Autodesk Inventor part; units mm, degrees
ref_plane "YZ Plane" through (0, 0, 0) normal (1, 0, 0) x (0, 1, 0)
ref_plane "XZ Plane" through (0, 0, 0) normal (0, 1, 0) x (-1, 0, 0)
ref_plane "XY Plane" through (0, 0, 0) normal (0, 0, 1) x (1, 0, 0)
sketch "Sketch1" plane through (0, 0, 0) normal (0, 0, 1) x (1, 0, 0)
  line L0 (-43.38, 0) -> (7.23, 0) construction
  line L1 (0, -97.41) -> (0, 25.51)
  line L2 (0, 7.95) -> (-31.775, 7.95)
  line L3 (-31.775, 7.95) -> (-31.775, 3.5363)
  line L4 (-31.775, 3.5363) -> (-28.125, 1.4289)
  line L5 (-28.125, 1.4289) -> (-28.125, -1.4289)
  line L6 (-31.775, -7.95) -> (0, -7.95)
  line L7 (-28.125, -1.4289) -> (-31.775, -3.5363)
  line L8 (-31.775, -3.5363) -> (-31.775, -7.95)
  circle A0 centre (-32.65, 0) radius 3.5 construction
  line L9 (-22.225, -7.95) -> (-22.225, -11.45)
  line L10 (-22.225, -11.45) -> (0, -11.45) construction
  line L11 (-22.225, -11.45) -> (-12.2465, -79.85)
  line L12 (-12.2465, -79.85) -> (-8, -79.85)
  line L13 (-8, -79.85) -> (-8, -54.85)
  line L14 (-8, -54.85) -> (0, -54.85)
  point P0 (0, 0)
  point P1 (-36.15, 0)
  dimension "d5" = 7
  dimension "d0" = 60
  dimension "d1" = 56.25
  dimension "d2" = 63.55
  dimension "d3" = 15.9
  dimension "d6" = 72.3
  dimension "d14" = 3.5
  dimension "d15" = 44.45
  dimension "d16" = 68.4
  dimension "d17" = 8.3
  dimension "d18" = 25
  dimension "d19" = 16
  dimension "d20" = 24.493
revolve "Revolution1" add sketch "Sketch1" angle 360 about axis through (0, -10, 0) along (0, 1, 0)
sketch "Sketch2" plane through (0, 7.95, 0) normal (0, 1, 0) x (1, 0, 0)
  circle A0 centre (0, 0) radius 31.775 construction
  line L0 (-44.485, 0) -> (44.485, 0) construction
  line L1 (0, 44.485) -> (0, -44.485) construction
  line L2 (-31.775, 8.05) -> (-23.825, 8.05)
  line L3 (-23.825, 8.05) -> (-23.825, -8.05)
  line L4 (-23.825, -8.05) -> (-31.775, -8.05)
  line L5 (-31.775, -8.05) -> (-31.775, 8.05)
  circle A1 centre (0, 0) radius 31.775
  line L6 (31.775, 8.05) -> (23.825, 8.05)
  line L7 (23.825, 8.05) -> (23.825, -8.05)
  line L8 (23.825, -8.05) -> (31.775, -8.05)
  line L9 (31.775, -8.05) -> (31.775, 8.05)
  point P0 (-31.775, 0)
  point P1 (31.775, 0)
  point P2 (30.7384, -8.05)
  point P3 (30.7384, 8.05)
  point P4 (-30.7384, 8.05)
  point P5 (-30.7384, -8.05)
  dimension "d12" = 16.1
  dimension "d13" = 47.65
extrude "Extrusion1" cut sketch "Sketch2" against normal through all contours L2 L3 L4 A1 | A1 L8 L7 L6
properties part number "SK40Collar"
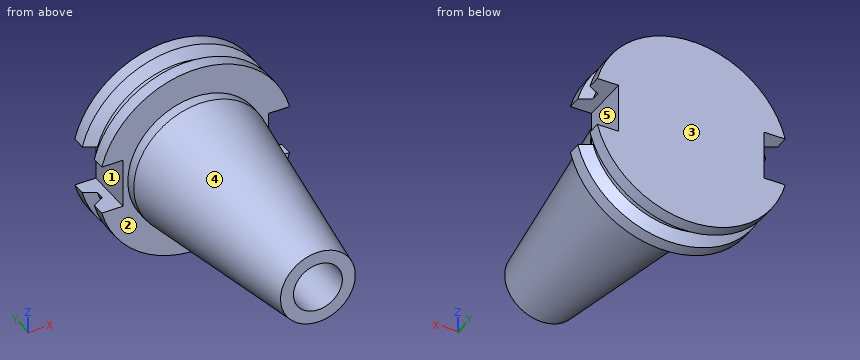
Build history of the part. All positions in model axes, mm. Face numbers are marked on the shaded views. A direction names the side the tool comes from. Give positions to 0.01 mm unless a question says otherwise; leave off trailing zeros. Loops run counter-clockwise (first coordinate to the right, second up) from the corner with the lowest first, then second, coordinate; pieces in that order, holes last.
1) Band-saw the part on C-C on y = -31. List the corners of the cut face in (x, z), then the cut area to 3 significant figures.
Values follow:
outline: circle Ø38.75 at (0, 0)
area: 1,180 mm2
2) Two-plate mould, pull along Z, no slides. Class the marked faces 3, 4 and 5: released by +Z, released by -Z, zero draft, split by the parting line, or undercut.
Values follow:
face 3: zero draft
face 4: split by the parting line
face 5: undercut
3) Band-saw the part on D-D on y = -45.5. List the corners of the cut face in (x, z).
Values follow:
outline: circle Ø34.52 at (0, 0)
4) Probe line 1 along Y through (x, z) = (23.5, 20.5); line 2 along X through (y, z) = (-72, 3); line 3 along Z through (x, y) = (0, -66.5). List the from-to ranges inside material, lowest first.
Values follow:
line 1: y = -7.95 to -3.2, 3.2 to 7.95
line 2: x = -13.05 to -7.42, 7.42 to 13.05
line 3: z = -14.19 to -8, 8 to 14.19
5) Drop flat-ended pins along their axis: P1, Ø21, axis at x = 0, z = 0, coming from the -Y side; P2, Ø7.5, axis at x = 27.5, y = 3.5, coming from the -Z side; P3, Ø8, axis at y = 1.5, z = 0, coming from the -X side (3 decimals); P4, Ø7.5, axis at x = 27, y = -1.5, coming from the +Z side. Give the stop position or say it passes through.
Values follow:
P1: stops at y = -79.85
P2: stops at z = -21.11
P3: stops at x = -23.825
P4: stops at z = 20.99
6) 3-axis set-ups, long thin cutter, end or side, ignore diameter. For the marked faces 1 and 2: which of +Z, -Z, +X, -X, +Y, -Y reach the whole face in a straight line?
Values follow:
face 1: -X, +Y, -Y
face 2: -Y
